```python
from build123d import *

# Parameters (mm, degrees)
BOSS_EXTRUDE1_DEPTH     = 12.3
BOSS_EXTRUDE1_2_DEPTH   = 12.3
SKETCH1_3_W             = 13
SKETCH1_3_H             = 23
BOSS_EXTRUDE2_DEPTH     = 1
BOSS_EXTRUDE3_START     = -12.3
BOSS_EXTRUDE3_OUTLINE_R = 0.946305397
BOSS_EXTRUDE3_DEPTH     = 12.3
CUT_EXTRUDE2_START      = -10.3
SKETCH1_6_R             = 0.946305397
CUT_EXTRUDE2_DEPTH      = 10.3
FILLET1_R               = 10
FILLET2_R               = 1.5


# Read off the part's stored shape, not the designer's step: Boss-Extrude3
with BuildPart() as part:
    # Sketch1 → Boss-Extrude1 (new body)
    with BuildSketch(Plane(origin=(0, 0, 0), x_dir=(1, 0, 0), z_dir=(0, 1, 0))):
        Polygon((10.5, 0), (9.7, 0), (9.7, -46.155014612), (10.5, -46.574062231), align=None)
    extrude(amount=-BOSS_EXTRUDE1_DEPTH)



with BuildPart() as body_2:
    # Sketch1 → Boss-Extrude1 2 (new body)
    with BuildSketch(Plane(origin=(0, 0, 0), x_dir=(1, 0, 0), z_dir=(0, 1, 0))):
        Polygon((-9.7, 0), (-10.5, 0), (-10.5, -35.574062231), (-9.7, -35.99310985), align=None)
    extrude(amount=-BOSS_EXTRUDE1_2_DEPTH)


with BuildPart() as part_1:
    add(part.part)

    add(body_2.part)  # Boss-Extrude2 merges body 2
    # Sketch1_3 → Boss-Extrude2 (add)
    with BuildSketch(Plane(origin=(0, 0, 0), x_dir=(1, 0, 0), z_dir=(0, 1, 0))):
        Polygon((9.7, 0), (-9.7, 0), (-9.7, -36.489905511), (-10.5, -36.489905511), (-10.5, -37.250622364), (10.5, -48.250622364), (10.5, -46.642015581), (9.7, -46.642015581), align=None)
        with Locations((0, -13.300665343)):
            Rectangle(SKETCH1_3_W, SKETCH1_3_H, mode=Mode.SUBTRACT)
    extrude(amount=-BOSS_EXTRUDE2_DEPTH)

    # Boss-Extrude3 outline → Boss-Extrude3 (add)
    with BuildSketch(Plane(origin=(0, 0, 0), x_dir=(1, 0, 0), z_dir=(0, 1, 0)).offset(BOSS_EXTRUDE3_START)):
        Polygon((-10.5, -45), (10.5, -56), (10.5, -46.574062231), (9.7, -46.155014612), (-9.7, -35.99310985), (-10.5, -35.574062231), align=None)
        with Locations((7.5, -52.5)):
            Circle(BOSS_EXTRUDE3_OUTLINE_R, mode=Mode.SUBTRACT)
        with Locations((-5.5, -43.7)):
            Circle(BOSS_EXTRUDE3_OUTLINE_R, mode=Mode.SUBTRACT)
    extrude(amount=BOSS_EXTRUDE3_DEPTH)

    # Sketch1_6 → Cut-Extrude2 (cut)
    # profile 1 of 3: a face of its own
    with BuildSketch(Plane(origin=(0, 0, 0), x_dir=(1, 0, 0), z_dir=(0, 1, 0)).offset(CUT_EXTRUDE2_START)):
        Polygon((10.5, -48.250622364), (-10.5, -37.250622364), (-10.5, -45), (10.5, -56), align=None)
        with Locations(Location((-5.5, -43.7, 0), (0, 0, 270))):
            Circle(SKETCH1_6_R, mode=Mode.SUBTRACT)
        with Locations(Location((7.5, -52.5, 0), (0, 0, 270))):
            Circle(SKETCH1_6_R, mode=Mode.SUBTRACT)
    # profile 2 of 3: a face of its own
    with BuildSketch(Plane(origin=(0, 0, 0), x_dir=(1, 0, 0), z_dir=(0, 1, 0)).offset(CUT_EXTRUDE2_START)):
        with Locations(Location((-5.5, -43.7, 0), (0, 0, 270))):
            Circle(SKETCH1_6_R)
    # profile 3 of 3: a face of its own
    with BuildSketch(Plane(origin=(0, 0, 0), x_dir=(1, 0, 0), z_dir=(0, 1, 0)).offset(CUT_EXTRUDE2_START)):
        with Locations(Location((7.5, -52.5, 0), (0, 0, 270))):
            Circle(SKETCH1_6_R)
    extrude(amount=CUT_EXTRUDE2_DEPTH, mode=Mode.SUBTRACT)

    # Fillet1
    fillet1_edges = [part_1.edges().sort_by_distance(p)[0] for p in [
        (-10.5, -11.3, 45),
    ]]
    fillet(fillet1_edges, radius=FILLET1_R)

    # Fillet2
    fillet2_edges = [part_1.edges().sort_by_distance(p)[0] for p in [
        (10.5, -6.15, 0),
        (10.5, -11.3, 56),
        (10.5, -5.15, 48.250622364),
        (-10.5, -6.15, 0),
        (-10.5, -5.15, 37.250622364),
    ]]
    fillet(fillet2_edges, radius=FILLET2_R)


solid = part_1.part
```
The model under review builds one solid part; all positions refer to its coordinate system, in mm. A direction names the side the tool comes from. Give positions to 0.01 mm unless a question says otherwise; leave off trailing zeros. Write each loop counter-clockwise with the first axis right and the second up, starting at its lowest first coordinate (ties: lowest second). Pieces come first, ordered by that corner, then holes.
(1) Consider section A-A, the plane z = 3. Give the boundary of the cut face in (x, y), and give its area (3 significant figures).
(2) Consider section B-B, the plane y = -7.5. Give the boundary of the cut face in (x, z).
(3) Consider section C-C, the plane x = 7.5. Give the boundary of the cut face in (y, z).
(4) For P1, Ø2, axis at x = 7.5, z = 52.5, coming from the +Y side; P2, Ø6, axis at x = 6, z = 49, coming from the +Y side; P3, Ø5, axis at x = 3.5, y = -10.5, coming from the -Z side, all flat-tipped, find the tip position at first contact; note any pin that passes through.
(5) To check wall thickness, follow L1, parallel to X at y = -5, z = 2; L2, parallel to X at y = -11.3, z = 43.7; L3, parallel to Y at x = 8.5, z = 34.5. State the ranges of each line that lie inside material, in increasing order.
(6) The part is to be moulded in two halves that separate along Z. For faces 1 (the cylindrical face through (10.238, -6.236, 0.653)), 2 (the flat face through (-6.5, -0.5, 13.5)), 3 (the cylindrical face through (-9.016, -11.286, 44.191)), say which applies: released by +Z, released by -Z, zero draft, split by the parting line, or undercut.
(7) Consider section D-D, the plane z = 52.5. Give the boundary of the cut face in (x, y), and give its area (3 significant figures).
(8) Tool access review of faces 4 (the flat face through (0, -1, 28)), 5 (the flat face through (0, 0, 29)), 6 (the flat face through (-0.1, -0.5, 24.801)), 7 (the cylindrical face through (-10.29, -5.08, 37.11)), 8 (the cylindrical face through (9.795, -5.078, 47.044)): name each direction out of +Z, -Z, +X, -X, +Y, -Y from which nothing blocks a thin tool from reaching the whole face with its end or side.
Returned:
1. outline: (-10.5, -12.3) - (-9.7, -12.3) - (-9.7, -1) - (-6.5, -1) - (-6.5, 0) - (-10.5, 0) - close; (6.5, -1) - (9.7, -1) - (9.7, -12.3) - (10.5, -12.3) - (10.5, 0) - (6.5, 0) - close
1. area: 26.1 mm2
2. outline: (-10.5, 1.5) arc R1.5 ccw to (-9.7, 0.17) - (-9.7, 35.99) - (9.7, 46.16) - (9.7, 0.17) arc R1.5 ccw to (10.5, 1.5) - (10.5, 45.77) arc R1.5 ccw to (8.3, 47.1) - (-9.7, 37.67) arc R1.5 ccw to (-10.5, 36.34) - close
3. outline: (-12.3, 45) - (-1, 45) - (-1, 0) - (0, 0) - (0, 46.68) - (-10.3, 46.68) - (-10.3, 51.55) - (-12.3, 51.55) - close; (-12.3, 53.45) - (-10.3, 53.45) - (-10.3, 54.43) - (-12.3, 54.43) - close
4. P1: stops at y = -10.3
4. P2: stops at y = 0
4. P3: stops at z = 41.6
5. L1: x = -10.5 to -9.7, 9.7 to 10.5
5. L2: x = -9.3 to -6.45, -4.55 to 5.01, 9.7 to 10.5
5. L3: y = -1 to 0
6. face 1: released by -Z
6. face 2: undercut
6. face 3: released by +Z
7. outline: (3.82, -12.3) - (6.55, -12.3) - (6.55, -10.3) - (3.82, -10.3) - close; (8.45, -12.3) - (10.5, -12.3) - (10.5, -10.3) - (8.45, -10.3) - close
7. area: 9.58 mm2
8. face 4: -Z, -Y
8. face 5: +Z, -Z, +X, -X, +Y
8. face 6: +Y, -Y
8. face 7: +Z, -X, +Y
8. face 8: +Z, +Y
